Autodesk Inventor part; units mm, degrees
ref_plane "YZ Plane" through (0, 0, 0) normal (1, 0, 0) x (0, 1, 0)
ref_plane "XZ Plane" through (0, 0, 0) normal (0, 1, 0) x (-1, 0, 0)
ref_plane "XY Plane" through (0, 0, 0) normal (0, 0, 1) x (1, 0, 0)
sketch "Sketch1" plane through (0, 0, 0) normal (0, 0, 1) x (1, 0, 0)
  line L0 (77.9423, 0) -> (38.9711, -67.5)
  line L1 (38.9711, -67.5) -> (-38.9711, -67.5)
  line L2 (-38.9711, -67.5) -> (-77.9423, 0)
  line L3 (-77.9423, 0) -> (-38.9711, 67.5)
  line L4 (-38.9711, 67.5) -> (38.9711, 67.5)
  line L5 (38.9711, 67.5) -> (77.9423, 0)
  circle A0 centre (0, 0) radius 12.5
  circle A1 centre (54, 0) radius 2.5
  circle A2 centre (46.7654, 27) radius 2.5
  circle A3 centre (27, 46.7654) radius 2.5
  circle A4 centre (0, 54) radius 2.5
  circle A5 centre (-27, 46.7654) radius 2.5
  circle A6 centre (-46.7654, 27) radius 2.5
  circle A7 centre (-54, 0) radius 2.5
  circle A8 centre (-46.7654, -27) radius 2.5
  circle A9 centre (-27, -46.7654) radius 2.5
  circle A10 centre (0, -54) radius 2.5
  circle A11 centre (27, -46.7654) radius 2.5
  circle A12 centre (46.7654, -27) radius 2.5
  dimension "d0" = 135
  dimension "d1" = 25
  dimension "d2" = 54
  dimension "d3" = 5
  dimension "d6" = 360
extrude "Extrusion1" add sketch "Sketch1" along normal blind 10
sketch "Sketch2" plane through (0, 0, 10) normal (0, 0, 1) x (1, 0, 0)
  circle A0 centre (0, 45) radius 2.5
  circle A1 centre (-45, 0) radius 2.5
  circle A2 centre (0, -45) radius 2.5
  circle A3 centre (45, 0) radius 2.5
  point P0 (0, 0)
  dimension "d10" = 5
  dimension "d11" = 45
  dimension "d14" = 360
extrude "Extrusion2" cut sketch "Sketch2" against normal through all contours A0 | A2
sketch "Sketch4" plane through (0, 0, 10) normal (0, 0, 1) x (1, 0, 0)
  circle A0 centre (0, 45) radius 2.5
  circle A1 centre (0, 45) radius 6.5
  circle A2 centre (-45, 0) radius 6.5
  circle A3 centre (0, -45) radius 6.5
  circle A4 centre (45, 0) radius 6.5
  point P0 (0, 0)
  dimension "d22" = 13
  dimension "d28" = 360
extrude "Extrusion4" cut sketch "Sketch4" against normal blind 5 contours A1 | A3
properties part number "AC04" material "ABS Plastic"
Geometry: final body of the model. Coordinates: model frame, mm. A direction names the side the tool comes from. Round coordinates to 2 decimals unless told otherwise and drop trailing zeros. Loops run counter-clockwise (first coordinate to the right, second up) from the corner with the lowest first, then second, coordinate; pieces in that order, holes last. Notation, with made-up numbers: (76, -23.75) -> (118, -23.75) arc R16 ccw to (118, -17.75) -> close; hole circle Ø7 at (-37.5, 39). An arc over 180 degrees is marked (long way). Use one line per item in the form item = value.
Item 1: Cut plane D-D on x = -54. Output: boundary loops of the cut face in (y, z), then the cut area to 3 significant figures.
Evaluation:
outline = (-41.47, 0) -> (-2.5, 0) -> (-2.5, 10) -> (-41.47, 10) -> close; (2.5, 0) -> (41.47, 0) -> (41.47, 10) -> (2.5, 10) -> close
area = 779 mm2
Item 2: Cut plane C-C on z = 8. Give the number of separate pieces and of enclosed holes in the cut face, then the cut area to 3 significant figures.
Evaluation:
separate_pieces = 1
enclosed_holes = 15
area = 14,800 mm2
Item 3: Cut plane A-A on x = 27. Output: boundary loops of the cut face in (y, z), then the cut area to 3 significant figures.
Evaluation:
outline = (-67.5, 0) -> (-49.27, 0) -> (-49.27, 10) -> (-67.5, 10) -> close; (-44.27, 0) -> (44.27, 0) -> (44.27, 10) -> (-44.27, 10) -> close; (49.27, 0) -> (67.5, 0) -> (67.5, 10) -> (49.27, 10) -> close
area = 1,250 mm2
Item 4: Cut plane B-B on y = -27. Output: boundary loops of the cut face in (x, z), then the cut area to 3 significant figures.
Evaluation:
outline = (-62.35, 0) -> (-49.27, 0) -> (-49.27, 10) -> (-62.35, 10) -> close; (-44.27, 0) -> (44.27, 0) -> (44.27, 10) -> (-44.27, 10) -> close; (49.27, 0) -> (62.35, 0) -> (62.35, 10) -> (49.27, 10) -> close
area = 1,150 mm2
Item 5: Access query for faces 1 (the cylindrical face through (25.157, 45.076, 4.93)), 2 (the flat face through (3, -45, 5)). Directions: +Z, -Z, +X, -X, +Y, -Y. A direction counts if a zero-diameter tool reaches every point of the face in a straight line with its end or side. Return the directions, or none.
Evaluation:
face_1 = +Z, -Z
face_2 = +Z
Item 6: Contact query for flat-ended pins moving along their axis: pin 1 Ø1 at (y, z) = (-7.5, 1.5) entering from +X; pin 2 Ø6.5 at (x, y) = (1.5, -46) entering from +Z; pin 3 Ø3 at (y, z) = (52, 6) entering from +X. Output: stop coordinate, or through.
Evaluation:
pin_1 = 73.9
pin_2 = 5
pin_3 = 48.79
Item 7: Draft query along X for faces 3 (the flat face through (-1, 67.5, 5)), 4 (the flat face through (58.73, -33.28, 4.93)), 5 (the cylindrical face through (49.15, 26.25, 4.93)), 6 (the flat face through (-58.73, 33.28, 4.93)). Return one class per face: released by +X, released by -X, zero draft, split by the parting line, or undercut.
Evaluation:
face_3 = zero draft
face_4 = released by +X
face_5 = undercut
face_6 = released by -X
Item 8: Material intervals for probe 1 along Y at (x, z) = (0, 3.55); probe 2 along Y at (x, z) = (-27, 5); probe 3 along X at (y, z) = (-26, 2.75), sorted ascending.
Evaluation:
probe_1 = -67.5 to -56.5, -51.5 to -47.5, -42.5 to -12.5, 12.5 to 42.5, 47.5 to 51.5, 56.5 to 67.5
probe_2 = -67.5 to -49.27, -44.27 to 44.27, 49.27 to 67.5
probe_3 = -62.93 to -49.06, -44.47 to 44.47, 49.06 to 62.93
